```python
from build123d import *
from build123d.topology import SkipClean

# Parameters (mm, degrees)
SKETCH1_R           = 7.5
SKETCH1_R_2         = 3.285
BOSS_EXTRUDE1_DEPTH = 2
SKETCH1_3_R         = 10
SKETCH1_3_R_2       = 7.5
BOSS_EXTRUDE2_DEPTH = 14
BOSS_EXTRUDE3_DEPTH = 10
BOSS_EXTRUDE4_DEPTH = 8
FILLET1_R           = 2
FILLET2_R           = 2
SKETCH4_W           = 2
SKETCH4_H           = 8
BOSS_EXTRUDE5_DEPTH = 15
CHAMFER1_SIZE       = 2
CUT_EXTRUDE1_REACH  = 55.102
SKETCH6_R           = 1.825
SKETCH7_W           = 2
SKETCH7_H           = 8
BOSS_EXTRUDE6_DEPTH = 6
CUT_EXTRUDE2_REACH  = 56.289
SKETCH8_R           = 1.825


with BuildPart() as part:
    # Sketch1 → Boss-Extrude1 (new body)
    with BuildSketch(Plane.XY):
        Circle(SKETCH1_R)
        Circle(SKETCH1_R_2, mode=Mode.SUBTRACT)
    extrude(amount=BOSS_EXTRUDE1_DEPTH)

    # Sketch1<3> → Boss-Extrude2 (add)
    with BuildSketch(Plane.XY):
        Circle(SKETCH1_3_R)
        Circle(SKETCH1_3_R_2, mode=Mode.SUBTRACT)
    extrude(amount=BOSS_EXTRUDE2_DEPTH)

    # Sketch2 → Boss-Extrude3 (add)
    with SkipClean():  # the faces are left unmerged after this step: merging them gives an invalid solid
        with BuildSketch(Plane.XY.offset(14)):
            with BuildLine():
                ThreePointArc((0.880723614, 9.961140794), (-9.097879067, 4.150734451), (-6.945976325, -7.193984493))
                Line((-6.945976325, -7.193984493), (-5.209482244, -5.39548837))
                ThreePointArc((-5.209482244, -5.39548837), (-6.8234093, 3.113050838), (0.66054271, 7.470855595))
                Line((0.66054271, 7.470855595), (0.880723614, 9.961140794))
            make_face()
            with BuildLine():
                Line((-0.66054271, -7.470855595), (-0.880723614, -9.961140794))
                ThreePointArc((-0.880723614, -9.961140794), (6.752509306, -7.375880833), (10, 0))
                ThreePointArc((10, 0), (9.204883575, 3.907699883), (6.945976325, 7.193984493))
                Line((6.945976325, 7.193984493), (5.209482244, 5.39548837))
                ThreePointArc((5.209482244, 5.39548837), (6.903662681, 2.930774912), (7.5, 0))
                ThreePointArc((7.5, 0), (5.06438198, -5.531910625), (-0.66054271, -7.470855595))
            make_face()
        extrude(amount=BOSS_EXTRUDE3_DEPTH)

    # Sketch3 → Boss-Extrude4 (add)
    with SkipClean():  # the faces are left unmerged after this step: merging them gives an invalid solid
        with BuildSketch(Plane.XY.offset(24)):
            Polygon((10.711806124, -12.659273659), (9.733468631, -14.80366432), (-17.56016857, -2.351460968), (-16.581831078, -0.207070307), align=None)
        extrude(amount=BOSS_EXTRUDE4_DEPTH)

    # Fillet1
    # the kernel refuses this fillet: 2 mm, written as the material it adds along each edge
    with BuildSketch(Plane(origin=(-5.209482244, -5.39548837, 24), x_dir=(0.4150734450654639, 0.9097879067131457, 0), z_dir=(0.9097879067131457, -0.41507344506546395, 0))) as fillet1_piece_1_section:
        with BuildLine():
            CenterArc((FILLET1_R, FILLET1_R), FILLET1_R, 180, 90)
            Line((0, FILLET1_R), (0, 0))
            Line((0, 0), (FILLET1_R, 0))
        make_face()
    fillet1_piece_1 = extrude(amount=14.571067812, mode=Mode.PRIVATE)
    fillet1_piece_1 = fillet1_piece_1 & Plane(origin=(0, 0, 24.466684855), x_dir=(-0.08807236135728662, -0.9961140793929938, 0), z_dir=(0, 0, -1)) * Cylinder(10, 38, mode=Mode.PRIVATE)
    fillet1_piece_1 = fillet1_piece_1 - Plane(origin=(0, 0, 24.466684855), x_dir=(0.6945976324993828, 0.7193984493493522, 0), z_dir=(0, 0, -1)) * Cylinder(7.5, 38, mode=Mode.PRIVATE)
    add(fillet1_piece_1)
    with BuildSketch(Plane(origin=(-13.917123993, -1.42279228, 24), x_dir=(0.4150734450654639, 0.9097879067131457, 0), z_dir=(0.9097879067131457, -0.41507344506546395, 0))) as fillet1_piece_2_section:
        with BuildLine():
            CenterArc((FILLET1_R, FILLET1_R), FILLET1_R, 180, 90)
            Line((0, FILLET1_R), (0, 0))
            Line((0, 0), (FILLET1_R, 0))
        make_face()
    fillet1_piece_2 = extrude(amount=14.571067812, mode=Mode.PRIVATE)
    fillet1_piece_2 = fillet1_piece_2 & Plane(origin=(0, 0, 24.466680249), x_dir=(0.08807236135728662, 0.9961140793929938, 0), z_dir=(0, 0, -1)) * Cylinder(10, 38, mode=Mode.PRIVATE)
    fillet1_piece_2 = fillet1_piece_2 - Plane(origin=(0, 0, 24.466680249), x_dir=(0.6945976324993828, 0.7193984493493522, 0), z_dir=(0, 0, -1)) * Cylinder(7.5, 38, mode=Mode.PRIVATE)
    add(fillet1_piece_2)

    # Fillet2
    # the kernel refuses this fillet: 2 mm, written as the material it adds along each edge
    with BuildSketch(Plane(origin=(0, 0, 24), x_dir=(-0.9898439357335846, 0.14215830222483344, 0), z_dir=(0.14215830222483344, 0.9898439357335846, 0))) as fillet2_piece_1_section:
        with BuildLine():
            CenterArc((10 + FILLET2_R, -FILLET2_R), FILLET2_R, 90, 90)
            Line((10 + FILLET2_R, 0), (10, 0))
            Line((10, 0), (10, -FILLET2_R))
        make_face()
    fillet2_piece_1 = revolve(axis=Axis((0, 0, 24), (0, 0, 1)), revolution_arc=82.826410261, mode=Mode.PRIVATE)
    fillet2_piece_1 = split(fillet2_piece_1, bisect_by=Plane(origin=(-8.477218422, -3.904645831, 23.537511225), z_dir=(-0.41507344506546395, -0.9097879067131457, 0)), keep=Keep.TOP, mode=Mode.PRIVATE)
    fillet2_piece_1 = split(fillet2_piece_1, bisect_by=Plane(origin=(-9.455555915, -6.049036492, 23.537511225), z_dir=(0.41507344506546395, 0.9097879067131456, 0)), keep=Keep.TOP, mode=Mode.PRIVATE)
    add(fillet2_piece_1)
    with BuildSketch(Plane(origin=(0, 0, 24), x_dir=(0.7561376391606037, -0.6544126149797455, 0), z_dir=(0.6544126149797455, 0.7561376391606037, 0))) as fillet2_piece_2_section:
        with BuildLine():
            CenterArc((10 + FILLET2_R, FILLET2_R), FILLET2_R, 180, 90)
            Line((10 + FILLET2_R, 0), (10, 0))
            Line((10, 0), (10, FILLET2_R))
        make_face()
    fillet2_piece_2 = revolve(axis=Axis((0, 0, 24), (0, 0, -1)), revolution_arc=82.826410261, mode=Mode.PRIVATE)
    fillet2_piece_2 = split(fillet2_piece_2, bisect_by=Plane(origin=(2.607194883, -8.96169878, 23.537511389), z_dir=(-0.41507344506546395, -0.9097879067131457, 0)), keep=Keep.TOP, mode=Mode.PRIVATE)
    fillet2_piece_2 = split(fillet2_piece_2, bisect_by=Plane(origin=(1.628857391, -11.106089441, 23.537511389), z_dir=(0.41507344506546395, 0.9097879067131456, 0)), keep=Keep.TOP, mode=Mode.PRIVATE)
    add(fillet2_piece_2)

    # Sketch4 → Boss-Extrude5 (add)
    with BuildSketch(Plane(origin=(-3.913349969, -8.577562644, 0), x_dir=(0.9097879067131455, -0.4150734450654641, 0), z_dir=(-0.4150734450654641, -0.9097879067131455, 0))):
        with Locations((-14, 28)):
            Rectangle(SKETCH4_W, SKETCH4_H)
        with Locations((14, 28)):
            Rectangle(SKETCH4_W, SKETCH4_H)
    extrude(amount=BOSS_EXTRUDE5_DEPTH)

    # Chamfer1
    chamfer1_edges = [part.edges().sort_by_distance(p)[0] for p in [
        (-15.740592757, -3.181607858, 28),
        (7.913892818, -13.97351743, 28),
    ]]
    chamfer(chamfer1_edges, length=CHAMFER1_SIZE)

    # Cut-Extrude1: up to this face of the body (flat: up to its plane)
    cut_extrude1_end = Plane(part.part.faces().sort_by_distance((7.10958654, -20.55487829, 28))[0])
    # Sketch6 → Cut-Extrude1 (cut, up to the picked face)
    with BuildSketch(Plane(origin=(-13.646818601, 6.226101676, 0), x_dir=(0, 0, 1), z_dir=(-0.9097879067131456, 0.41507344506546384, 0)), mode=Mode.PRIVATE) as cut_extrude1_sk1:
        with Locations(Location((28, -21.428090416, 0), (0, 0, 270))):
            Circle(SKETCH6_R)
    cut_extrude1_tool1 = split(extrude(cut_extrude1_sk1.sketch, amount=-CUT_EXTRUDE1_REACH, mode=Mode.PRIVATE), bisect_by=cut_extrude1_end, keep=Keep.BOTH, mode=Mode.PRIVATE)
    add(cut_extrude1_tool1.solids().sort_by(Axis((-22.54105, -13.268916, 28), (0.9097879067131456, -0.41507344506546384, 0)))[0], mode=Mode.SUBTRACT)

    # Sketch7 → Boss-Extrude6 (add)
    with BuildSketch(Plane(origin=(-2.935012477, -6.433171983, 0), x_dir=(0.9097879067131457, -0.4150734450654639, 0), z_dir=(0.41507344506546384, 0.9097879067131456, 0))):
        with Locations((14, -28)):
            Rectangle(SKETCH7_W, SKETCH7_H)
        with Locations((-14, -28)):
            Rectangle(SKETCH7_W, SKETCH7_H)
    extrude(amount=BOSS_EXTRUDE6_DEPTH)

    # Cut-Extrude2: up to this face of the body (flat: up to its plane)
    cut_extrude2_end = Plane(part.part.faces().sort_by_distance((7.301672081, -20.133851349, 28))[0])
    # Sketch8 → Cut-Extrude2 (cut, up to the picked face)
    with BuildSketch(Plane(origin=(-13.646818601, 6.226101676, 0), x_dir=(0, 0, 1), z_dir=(-0.9097879067131456, 0.4150734450654639, 0)), mode=Mode.PRIVATE) as cut_extrude2_sk1:
        with Locations(Location((28, -4.428090416, 0), (0, 0, 270))):
            Circle(SKETCH8_R)
    cut_extrude2_tool1 = split(extrude(cut_extrude2_sk1.sketch, amount=-CUT_EXTRUDE2_REACH, mode=Mode.PRIVATE), bisect_by=cut_extrude2_end, keep=Keep.BOTH, mode=Mode.PRIVATE)
    add(cut_extrude2_tool1.solids().sort_by(Axis((-15.484801, 2.197479, 28), (0.9097879067131456, -0.4150734450654639, 0)))[0], mode=Mode.SUBTRACT)


solid = part.part
```
Geometry check sheet. Reference: the model listing, model coordinates, mm. A direction names the side the tool comes from. Round coordinates to 2 decimals unless told otherwise and drop trailing zeros. Order: outer loops, then holes, each group sorted by start corner. A loop starts at its lowest first (then second) coordinate and runs counter-clockwise, first axis right, second up. Notation, with made-up numbers: (49, 20.25) - (59, 20.25) arc R7 cw to (59, 32.25) - close; hole circle Ø8 at (19, 33). An arc over 180 degrees is marked (long way). Use a Markdown table: item, result. Add a question column.
1) Thickness scan on line 1 along Y through (x, z) = (0, 1.4) (3 decimals); line 2 along X through (y, z) = (0, 11.5). Record the ranges inside material, lowest first.
2) Section check A-A (z = 18.5). Record the cut outline in (x, y).
3) Gauge pin test, flat ends, axial feed: P1, Ø2.5, axis at x = 2, y = 8, coming from the +Z side; P2, Ø12, axis at x = -0.5, y = 3.5, coming from the +Z side; P3, Ø8, axis at y = -1.5, z = 22, coming from the +X side. Record the tip position at first contact, or that the pin passes through.
4) Section check B-B (z = 27.5). Count the separate pieces of the cut face and the enclosed holes in it, then the cut area to 3 significant figures.
5) Mould release check, pull along Y, two halves, no side actions. Record for faces 4 (the flat face through (0.77, 8.7, 18.93)), 5 (the flat face through (-17, -5, 24)), 6 (the flat face through (-19.23, -10.83, 27.94)), 7 (the flat face through (-0.77, -8.7, 18.93)): released by +Y, released by -Y, zero draft, split by the parting line, or undercut.
6) Section check C-C (z = 4.5). Record the cut outline in (x, y).
7) Set-up check for faces 1 (the flat face through (-13.26, 2.26, 29.83)), 2 (the flat face through (-6.09, -6.31, 18.93)), 3 (the flat face through (6.6, -14.5, 27.9)): record each of +Z, -Z, +X, -X, +Y, -Y from which the full face is reachable in a straight line by a thin tool's end or side.
Established:
| question | item | result |
|---|---|---|
| 1 | line 1 | -10 to -3.285, 3.285 to 10 |
| 1 | line 2 | -10 to -7.5, 7.5 to 10 |
| 2 | outline | (-6.95, -7.19) - (-5.21, -5.4) arc R7.5 cw to (0.66, 7.47) - (0.88, 9.96) arc R10 ccw to start; (-0.88, -9.96) arc R10 ccw to (6.95, 7.19) - (5.21, 5.4) arc R7.5 cw to (-0.66, -7.47) - close |
| 3 | P1 | z = 14 |
| 3 | P2 | z = 24 |
| 3 | P3 | x = 10 |
| 4 | separate pieces | 5 |
| 4 | enclosed holes | 0 |
| 4 | area | 131 mm2 |
| 5 | face 4 | undercut |
| 5 | face 5 | zero draft |
| 5 | face 6 | released by -Y |
| 5 | face 7 | undercut |
| 6 | outline | circle Ø20 at (0, 0); hole circle Ø15 at (0, 0) |
| 7 | face 1 | +Z, -Z, +X |
| 7 | face 2 | -Y |
| 7 | face 3 | +Z, -Z |
